Part model, mm, in its own coordinate system. Face numbers are marked on the shaded views. A direction names the side the tool comes from. Give positions to 0.01 mm unless a question says otherwise; leave off trailing zeros. Order: outer loops, then holes, each group sorted by start corner. A loop starts at its lowest first (then second) coordinate and runs counter-clockwise, first axis right, second up. Notation, with made-up numbers: M -9,-34.75 L 18,-34.75 A19 cw 18,-7.75 Z; hole C 49,59.5 d6. An arc over 180 degrees is marked long. Return JSON: item names as keys, results as strings.
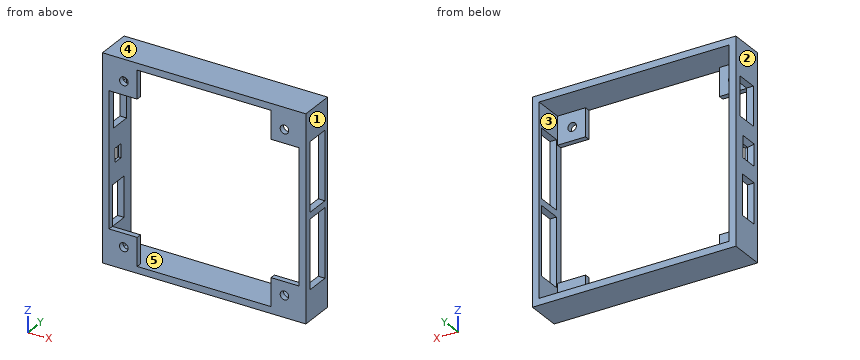
from build123d import *

# Parameters (mm, degrees)
SKETCH_1_W                  = 76
SKETCH_1_H                  = 76
EXTRUDE_1_DEPTH             = 13
SKETCH_2_W                  = 71
SKETCH_2_H                  = 71
CUT_EXTRUDE_1_DEPTH         = 11
SKETCH_3_R                  = 1.6
CUT_EXTRUDE_2_DEPTH         = 55.854352608
PATTERN_LINEAR_1_COUNT      = 2
PATTERN_LINEAR_1_PITCH      = 60
PATTERN_LINEAR_1_COUNT_DIR2 = 2
PATTERN_LINEAR_1_PITCH_DIR2 = 60
CUT_EXTRUDE_3_DEPTH         = 55.854352608
CUT_EXTRUDE_5_REACH         = 87.959
SKETCH_5_W                  = 14.5
SKETCH_5_H                  = 7.9
CUT_EXTRUDE_6_REACH         = 87.959
SKETCH_7_W                  = 25.542842713
SKETCH_7_H                  = 8.882842713
CUT_EXTRUDE_7_REACH         = 85.757
SKETCH_8_W                  = 5.1
SKETCH_8_H                  = 3.6
CUT_EXTRUDE_8_REACH         = 85.757
SKETCH_9_W                  = 15
SKETCH_9_H                  = 7
CHAMFER_1_SIZE              = 1.5


with BuildPart() as part:
    # 草图1 → 凸台-拉伸1 (new body)
    with BuildSketch(Plane(origin=(0, 0, 0), x_dir=(1, 0, 0), z_dir=(0, 1, 0))):
        Rectangle(SKETCH_1_W, SKETCH_1_H)
    extrude(amount=EXTRUDE_1_DEPTH)

    # 草图2 → 切除-拉伸1 (cut)
    with BuildSketch(Plane(origin=(0, 13, 0), x_dir=(1, 0, 0), z_dir=(0, 1, 0))):
        Rectangle(SKETCH_2_W, SKETCH_2_H)
    extrude(amount=-CUT_EXTRUDE_1_DEPTH, mode=Mode.SUBTRACT)

    # 草图3 → 切除-拉伸2 (cut, through all)
    with BuildSketch(Plane(origin=(0, 2, 0), x_dir=(1, 0, 0), z_dir=(0, 1, 0))):
        with Locations(Location((-30, 30, 0), (0, 0, 270))):
            Circle(SKETCH_3_R)
    cut_extrude_2 = extrude(amount=-CUT_EXTRUDE_2_DEPTH, mode=Mode.SUBTRACT)

    # 阵列(线性)1: Cut-Extrude 2 2 × 2
    with Locations(*[(i * PATTERN_LINEAR_1_PITCH, 0, j * PATTERN_LINEAR_1_PITCH_DIR2) for i in range(PATTERN_LINEAR_1_COUNT) for j in range(PATTERN_LINEAR_1_COUNT_DIR2) if (i, j) != (0, 0)]):
        add(cut_extrude_2, mode=Mode.SUBTRACT)

    # 草图4 → 切除-拉伸3 (cut, through all)
    with BuildSketch(Plane(origin=(0, 2, 0), x_dir=(1, 0, 0), z_dir=(0, 1, 0))):
        Polygon((35.5, -25), (25, -25), (25, -35.5), (-25, -35.5), (-25, -25), (-35.5, -25), (-35.5, 25), (-25, 25), (-25, 35.5), (25, 35.5), (25, 25), (35.5, 25), align=None)
    extrude(amount=-CUT_EXTRUDE_3_DEPTH, mode=Mode.SUBTRACT)

    # 草图5 → 切除-拉伸5 (cut, up to next)
    with BuildSketch(Plane.ZY.offset(38), mode=Mode.PRIVATE) as cut_extrude_5_sk1:
        with Locations((17.50009652, 6.536156877)):
            Rectangle(SKETCH_5_W, SKETCH_5_H)
    cut_extrude_5_tool1 = extrude(cut_extrude_5_sk1.sketch, amount=-CUT_EXTRUDE_5_REACH, mode=Mode.PRIVATE) & part.part
    add(cut_extrude_5_tool1.solids().sort_by_distance((-38, 6.536157, 17.500097))[0], mode=Mode.SUBTRACT)

    # 草图7 → 切除-拉伸6 (cut, up to next)
    with BuildSketch(Plane(origin=(38, 0, 0), x_dir=(0, 0, -1), z_dir=(1, 0, 0)), mode=Mode.PRIVATE) as cut_extrude_6_sk1:
        with Locations((13.99984252, 6.98615625)):
            Rectangle(SKETCH_7_W, SKETCH_7_H)
    cut_extrude_6_tool1 = extrude(cut_extrude_6_sk1.sketch, amount=-CUT_EXTRUDE_6_REACH, mode=Mode.PRIVATE) & part.part
    # 草图7 → 切除-拉伸6 (cut, up to next)
    with BuildSketch(Plane(origin=(38, 0, 0), x_dir=(0, 0, -1), z_dir=(1, 0, 0)), mode=Mode.PRIVATE) as cut_extrude_6_sk2:
        with Locations((-14.000215901, 6.98615625)):
            Rectangle(SKETCH_7_W, SKETCH_7_H)
    cut_extrude_6_tool2 = extrude(cut_extrude_6_sk2.sketch, amount=-CUT_EXTRUDE_6_REACH, mode=Mode.PRIVATE) & part.part
    add(cut_extrude_6_tool1.solids().sort_by_distance((38, 6.986156, -13.999843))[0], mode=Mode.SUBTRACT)
    add(cut_extrude_6_tool2.solids().sort_by_distance((38, 6.986156, 14.000216))[0], mode=Mode.SUBTRACT)

    # 草图8 → 切除-拉伸7 (cut, up to next)
    with BuildSketch(Plane(origin=(-35.5, 0, 0), x_dir=(0, 0, -1), z_dir=(1, 0, 0)), mode=Mode.PRIVATE) as cut_extrude_7_sk1:
        with Locations((-3.556e-05, 5.336156974)):
            Rectangle(SKETCH_8_W, SKETCH_8_H)
    cut_extrude_7_tool1 = extrude(cut_extrude_7_sk1.sketch, amount=-CUT_EXTRUDE_7_REACH, mode=Mode.PRIVATE) & part.part
    add(cut_extrude_7_tool1.solids().sort_by_distance((-35.5, 5.336157, 3.6e-05))[0], mode=Mode.SUBTRACT)

    # 草图9 → 切除-拉伸8 (cut, up to next)
    with BuildSketch(Plane(origin=(-35.5, 0, 0), x_dir=(0, 0, -1), z_dir=(1, 0, 0)), mode=Mode.PRIVATE) as cut_extrude_8_sk1:
        with Locations((17.5, 5.5)):
            Rectangle(SKETCH_9_W, SKETCH_9_H)
    cut_extrude_8_tool1 = extrude(cut_extrude_8_sk1.sketch, amount=-CUT_EXTRUDE_8_REACH, mode=Mode.PRIVATE) & part.part
    add(cut_extrude_8_tool1.solids().sort_by_distance((-35.5, 5.5, -17.5))[0], mode=Mode.SUBTRACT)

    # 倒角1
    chamfer_1_edges = [part.edges().sort_by_distance(p)[0] for p in [
        (-38, 5.336156974, -2.54996444),
        (-38, 3.536156974, 3.556e-05),
        (-38, 5.336156974, 2.55003556),
        (-38, 7.136156974, 3.556e-05),
    ]]
    chamfer(chamfer_1_edges, length=CHAMFER_1_SIZE)


solid = part.part
Q1. Pin check, flat tips, straight feed: pin 1 (5 mm diameter, centred on x = -31.5, z = 28, fed in from +Y); pin 2 (5 mm diameter, centred on x = -23, z = 26.5, fed in from -Y). Stop position of each tip, or through.
Established:
{"pin 1": "stops at y = 2", "pin 2": "stops at y = 0"}
Q2. 3-axis set-ups, long thin cutter, end or side, ignore diameter. For the marked faces 4 and 5: which of +Z, -Z, +X, -X, +Y, -Y reach the whole face in a straight line?
Established:
{"face 4": "+Z, +X, -X, +Y, -Y", "face 5": "+Y"}
Q3. Two-plate mould, pull along X, no slides. Class the marked faces 1, 2 and 3: +X half, -X half, draft (parallel to the pull), parting line (faces both ways), or undercut.
Established:
{"face 1": "+X half", "face 2": "-X half", "face 3": "undercut"}
Q4. Band-saw the part on A-A (x = 30). Give the cut face in (y, z).
Established:
{"outline": "M 0,-38 L 13,-38 L 13,-35.5 L 2,-35.5 L 2,-31.6 L 0,-31.6 Z; M 0,-28.4 L 2,-28.4 L 2,-25 L 0,-25 Z; M 0,25 L 2,25 L 2,28.4 L 0,28.4 Z; M 0,31.6 L 2,31.6 L 2,35.5 L 13,35.5 L 13,38 L 0,38 Z"}
Q5. Band-saw the part on C-C (x = 8.5). Give the cut face in (y, z).
Established:
{"outline": "M 0,-38 L 13,-38 L 13,-35.5 L 0,-35.5 Z; M 0,35.5 L 13,35.5 L 13,38 L 0,38 Z"}
Q6. Band-saw the part on B-B (z = -30). Give the cut face in (x, y), then the cut area to 3 significant figures.
Established:
{"outline": "M -38,0 L -31.6,0 L -31.6,2 L -35.5,2 L -35.5,13 L -38,13 Z; M -28.4,0 L -25,0 L -25,2 L -28.4,2 Z; M 25,0 L 28.4,0 L 28.4,2 L 25,2 Z; M 31.6,0 L 38,0 L 38,13 L 35.5,13 L 35.5,2 L 31.6,2 Z", "area": "94.2 mm²"}
Q7. Band-saw the part on D-D (z = -22). Give the cut face in (x, y).
Established:
{"outline": "M -38,0 L -35.5,0 L -35.5,2 L -38,2 Z; M -38,9 L -35.5,9 L -35.5,13 L -38,13 Z; M 35.5,0 L 38,0 L 38,2.54 L 35.5,2.54 Z; M 35.5,11.43 L 38,11.43 L 38,13 L 35.5,13 Z"}
Q8. Probe line 1 along X through (y, z) = (1.2, 30); line 2 along Z through (x, y) = (-27.5, 12.5). List the from-to ranges inside material, lowest first.
Established:
{"line 1": "x = -38 to -31.6, -28.4 to -25, 25 to 28.4, 31.6 to 38", "line 2": "z = -38 to -35.5, 35.5 to 38"}
